For this review, take the finished solid that the model builds, in its own axes (mm). A direction names the side the tool comes from. Coordinates: 2 decimals unless noted, no trailing zeros. Loops run counter-clockwise (first coordinate to the right, second up) from the corner with the lowest first, then second, coordinate; pieces in that order, holes last. Notation, with made-up numbers: (-36, 80) - (-24, 80) arc R27 cw to (-24, 105) - close; hole circle Ø5 at (33, 18). An arc over 180 degrees is marked (long way). One line per item, written item: value. Start each with the question number.
1. Take a section at C-C, the plane x = 5.5. State the section outline as (y, z) points, and give its area (3 significant figures).
2. For faces 4 (the face through (0, 29, 70)), 5 (the face through (-52, 21, 37)), 6 (the face through (0.09, 28.52, 37.95)), list the 3-axis set-ups (+Z, -Z, +X, -X, +Y, -Y) from which the entire face can be reached by the end or side of a thin tool; tool diameter is ignored.
3. Take a section at B-B, the plane z = 25.5. State the section outline as (x, y) points, and give its area (3 significant figures).
4. The part is to be moulded in two halves that separate along Z. For faces 1 (the face through (-32.967, 28.521, 39.733)), 2 (the face through (58, 29, 36)), 3 (the face through (-1, 0, 0)), say which applies: released by +Z, released by -Z, zero draft, split by the parting line, or undercut.
5. Take a section at A-A, the plane x = -35. State the section outline as (y, z) points.
6. Take a section at D-D, the plane y = -6.5. State the section outline as (x, z) points, and give its area (3 significant figures).
7. To check wall thickness, follow line 1 (X direction, y = -10, z = 48); line 2 (Y direction, x = 44, z = 39); line 3 (Y direction, x = 55, z = 59.25). State the ranges of each line that lie inside material, in increasing order. Write a range as from..to.
8. Insertion check: pin 1 (16 mm diameter, centred on x = 43, y = -18, fed in from +Z); pin 2 (1.3 mm diameter, centred on x = -55, y = 25.5, fed in from +Z); pin 3 (2.5 mm diameter, centred on x = 0, z = 40, fed in from +Y). Each pin has a flat end and moves straight along its axis. Give the tip position at first contact, or say it passes through.
```python
from build123d import *

# Parameters (mm, degrees)
SKETCH1_W           = 120
SKETCH1_H           = 60
BOSS_EXTRUDE1_DEPTH = 70
SKETCH2_W           = 114
SKETCH2_H           = 54
CUT_EXTRUDE1_DEPTH  = 67
FILLET3_R           = 5
FILLET4_R           = 2
SKETCH4_R           = 5
BOSS_EXTRUDE3_DEPTH = 67
FILLET5_R           = 2
SKETCH5_R           = 1.3
CUT_EXTRUDE2_DEPTH  = 18
SKETCH6_R           = 2.05
CUT_EXTRUDE3_DEPTH  = 3
CHAMFER2_SIZE       = 1
SKETCH7_R           = 6.25
CUT_EXTRUDE4_DEPTH  = 97.953597148
SKETCH8_R           = 8.75
CUT_EXTRUDE5_DEPTH  = 1.5


with BuildPart() as part:
    # Sketch1 → Boss-Extrude1 (new body)
    with BuildSketch(Plane.XY):
        Rectangle(SKETCH1_W, SKETCH1_H)
    extrude(amount=BOSS_EXTRUDE1_DEPTH)

    # Sketch2 → Cut-Extrude1 (cut)
    with BuildSketch(Plane.XY.offset(70)):
        Rectangle(SKETCH2_W, SKETCH2_H)
    extrude(amount=-CUT_EXTRUDE1_DEPTH, mode=Mode.SUBTRACT)

    # Fillet3
    fillet3_edges = [part.edges().sort_by_distance(p)[0] for p in [
        (60, -30, 35),
        (-60, -30, 35),
        (-60, 30, 35),
        (60, 30, 35),
    ]]
    fillet(fillet3_edges, radius=FILLET3_R)

    # Fillet4
    fillet4_edges = [part.edges().sort_by_distance(p)[0] for p in [
        (57, 27, 36.5),
        (57, -27, 36.5),
        (-57, -27, 36.5),
        (-57, 27, 36.5),
    ]]
    fillet(fillet4_edges, radius=FILLET4_R)

    # Sketch4 → Boss-Extrude3 (add)
    with BuildSketch(Plane.XY.offset(70)):
        with Locations((-55, 25)):
            Circle(SKETCH4_R)
        with Locations((55, 25)):
            Circle(SKETCH4_R)
        with Locations((55, -25)):
            Circle(SKETCH4_R)
        with Locations((-55, -25)):
            Circle(SKETCH4_R)
    extrude(amount=-BOSS_EXTRUDE3_DEPTH)

    # Fillet5
    fillet5_edges = [part.edges().sort_by_distance(p)[0] for p in [
        (-50.417424305, -27, 36.5),
        (-57, -20.417424305, 36.5),
        (57, -20.417424305, 36.5),
        (50.417424305, -27, 36.5),
        (50.417424305, 27, 36.5),
        (57, 20.417424305, 36.5),
        (-57, 20.417424305, 36.5),
        (-50.417424305, 27, 36.5),
    ]]
    fillet(fillet5_edges, radius=FILLET5_R)

    # Sketch5 → Cut-Extrude2 (cut)
    with BuildSketch(Plane.XY.offset(70)):
        with Locations((-55, 25)):
            Circle(SKETCH5_R)
        with Locations((55, 25)):
            Circle(SKETCH5_R)
        with Locations((55, -25)):
            Circle(SKETCH5_R)
        with Locations((-55, -25)):
            Circle(SKETCH5_R)
    extrude(amount=-CUT_EXTRUDE2_DEPTH, mode=Mode.SUBTRACT)

    # Sketch6 → Cut-Extrude3 (cut)
    with BuildSketch(Plane(origin=(0, 30, 0), x_dir=(1, 0, 0), z_dir=(0, 1, 0))):
        with Locations(Location((0, -40, 0), (0, 0, 270))):
            Circle(SKETCH6_R)
        with Locations(Location((35, -40, 0), (0, 0, 270))):
            Circle(SKETCH6_R)
        with Locations(Location((-35, -40, 0), (0, 0, 270))):
            Circle(SKETCH6_R)
    extrude(amount=-CUT_EXTRUDE3_DEPTH, mode=Mode.SUBTRACT)

    # Chamfer2
    chamfer2_edges = [part.edges().sort_by_distance(p)[0] for p in [
        (0, -30, 0),
        (60, 0, 0),
        (-60, 0, 0),
        (0, 30, 0),
        (-58.535533906, 28.535533906, 0),
        (58.535533906, 28.535533906, 0),
        (58.535533906, -28.535533906, 0),
        (-58.535533906, -28.535533906, 0),
    ]]
    chamfer(chamfer2_edges, length=CHAMFER2_SIZE)

    # Sketch7 → Cut-Extrude4 (cut, through all)
    with BuildSketch(Plane(origin=(0, 0, 0), x_dir=(-1, 0, 0), z_dir=(0, 0, -1))):
        with Locations((-43, -18)):
            Circle(SKETCH7_R)
    extrude(amount=-CUT_EXTRUDE4_DEPTH, mode=Mode.SUBTRACT)

    # Sketch8 → Cut-Extrude5 (cut)
    with BuildSketch(Plane.XY.offset(3)):
        with Locations((43, -18)):
            Circle(SKETCH8_R)
    extrude(amount=-CUT_EXTRUDE5_DEPTH, mode=Mode.SUBTRACT)


solid = part.part
```
Solutions:
1. outline: (-30, 1) - (-29, 0) - (29, 0) - (30, 1) - (30, 70) - (27, 70) - (27, 3) - (-27, 3) - (-27, 70) - (-30, 70) - close
1. area: 581 mm2
2. face 4: +Z, +X, -X, +Y, -Y
2. face 5: +Z
2. face 6: +Y
3. outline: (-60, -25) arc R5 ccw to (-55, -30) - (55, -30) arc R5 ccw to (60, -25) - (60, 25) arc R5 ccw to (55, 30) - (-55, 30) arc R5 ccw to (-60, 25) - close; hole (-57, -18) arc R2 ccw to (-55, -20) arc R5 cw to (-50, -25) arc R2 ccw to (-48, -27) - (48, -27) arc R2 ccw to (50, -25) arc R5 cw to (55, -20) arc R2 ccw to (57, -18) - (57, 18) arc R2 ccw to (55, 20) arc R5 cw to (50, 25) arc R2 ccw to (48, 27) - (-48, 27) arc R2 ccw to (-50, 25) arc R5 cw to (-55, 20) arc R2 ccw to (-57, 18) - close
3. area: 1,200 mm2
4. face 1: undercut
4. face 2: zero draft
4. face 3: released by -Z
5. outline: (-30, 1) - (-29, 0) - (29, 0) - (30, 1) - (30, 37.95) - (27, 37.95) - (27, 3) - (-27, 3) - (-27, 70) - (-30, 70) - close; (27, 42.05) - (30, 42.05) - (30, 70) - (27, 70) - close
6. outline: (-60, 1) - (-59, 0) - (59, 0) - (60, 1) - (60, 70) - (57, 70) - (57, 3) - (-57, 3) - (-57, 70) - (-60, 70) - close
6. area: 761 mm2
7. line 1: -60..-57, 57..60
7. line 2: -30..-27, 27..30
7. line 3: -30..-26.3, -23.7..-20, 20..23.7, 26.3..30
8. pin 1: z = 1.5
8. pin 2: z = 52
8. pin 3: y = -27
